```python
from build123d import *

# Parameters (mm, degrees)
SKETCH_1_R                       = 4
EXTRUDE_1_DEPTH                  = 41.5
HOLE_WIZARD_M4_1_D               = 3.3
HOLE_WIZARD_M4_1_DEPTH           = 12.1
HOLE_WIZARD_M4_1_TIP             = 0.991420021
HOLE_WIZARD_M4_1_ON_FACE_2_D     = 3.3
HOLE_WIZARD_M4_1_ON_FACE_2_DEPTH = 12.1
HOLE_WIZARD_M4_1_ON_FACE_2_TIP   = 0.991420021
CHAMFER_1_SIZE                   = 0.5
SKETCH_3_R                       = 2.5
EXTRUDE_1_2_DEPTH                = 6
CHAMFER_2_SIZE                   = 0.5
SKETCH_4_OUTSIDE_W               = 27.944
SKETCH_4_OUTSIDE_H               = 27.944
SKETCH_4_OUTSIDE_W_2             = 7
SKETCH_4_OUTSIDE_H_2             = 10.356925226
CUT_EXTRUDE_1_DEPTH              = 10


with BuildPart() as part:
    # 草图1 → Extrude 1 (new, symmetric)
    with BuildSketch(Plane.XY):
        Circle(SKETCH_1_R)
    extrude(amount=EXTRUDE_1_DEPTH, both=True)

    # M4 螺纹孔1
    with Locations(Plane.XY.offset(41.5)):
        with Locations((0, 0)):
            Hole(HOLE_WIZARD_M4_1_D / 2, depth=HOLE_WIZARD_M4_1_DEPTH)
            with Locations((0, 0, -(HOLE_WIZARD_M4_1_DEPTH + HOLE_WIZARD_M4_1_TIP / 2))):  # 118° drill point
                Cone(0, HOLE_WIZARD_M4_1_D / 2, HOLE_WIZARD_M4_1_TIP, mode=Mode.SUBTRACT)

    # M4 螺纹孔1 on face 2
    with Locations(Plane(origin=(0, 0, -41.5), x_dir=(-1, 0, 0), z_dir=(0, 0, -1))):
        with Locations((0, 0)):
            Hole(HOLE_WIZARD_M4_1_ON_FACE_2_D / 2, depth=HOLE_WIZARD_M4_1_ON_FACE_2_DEPTH)
            with Locations((0, 0, -(HOLE_WIZARD_M4_1_ON_FACE_2_DEPTH + HOLE_WIZARD_M4_1_ON_FACE_2_TIP / 2))):  # 118° drill point
                Cone(0, HOLE_WIZARD_M4_1_ON_FACE_2_D / 2, HOLE_WIZARD_M4_1_ON_FACE_2_TIP, mode=Mode.SUBTRACT)

    # 倒角1
    chamfer_1_edges = [part.edges().sort_by_distance(p)[0] for p in [
        (-4, 0, -41.5),
        (-4, 0, 41.5),
        (-1.65, 0, -41.5),
        (1.65, 0, 41.5),
    ]]
    chamfer(chamfer_1_edges, length=CHAMFER_1_SIZE)

    # 草图3 → Extrude 1 2 (add)
    with BuildSketch(Plane(origin=(0, 0, -41.5), x_dir=(-1, 0, 0), z_dir=(0, 0, -1))):
        with Locations(Location((0, 0, 0), (0, 0, 180))):
            Circle(SKETCH_3_R)
    extrude(amount=EXTRUDE_1_2_DEPTH)

    # 倒角2
    chamfer_2_edges = [part.edges().sort_by_distance(p)[0] for p in [
        (-2.5, 0, -47.5),
    ]]
    chamfer(chamfer_2_edges, length=CHAMFER_2_SIZE)

    # 草图4 outside → 切除-拉伸1 (cut)
    with BuildSketch(Plane(origin=(0, 0, -41.5), x_dir=(-1, 0, 0), z_dir=(0, 0, -1))):
        Rectangle(SKETCH_4_OUTSIDE_W, SKETCH_4_OUTSIDE_H)
        Rectangle(SKETCH_4_OUTSIDE_W_2, SKETCH_4_OUTSIDE_H_2, mode=Mode.SUBTRACT)
    extrude(amount=-CUT_EXTRUDE_1_DEPTH, mode=Mode.SUBTRACT)


solid = part.part
```
Check sheet for the modelled part. Datum: model origin and axes. Units: mm. A direction names the side the tool comes from. Give positions to 0.01 mm unless a question says otherwise; leave off trailing zeros. Write each loop counter-clockwise with the first axis right and the second up, starting at its lowest first coordinate (ties: lowest second). Pieces come first, ordered by that corner, then holes. Notation, with made-up numbers: (42.25, 50.25) -> (70.25, 50.25) arc R13 cw to (70.25, 64.25) -> close; hole circle Ø3 at (17, -36.75). An arc over 180 degrees is marked (long way). Use CSV: the item, a comma, the result in double quotes. Start each with the question number.
Q1. Tool access check on faces 1 (the flat face through (2, -2, -41.5)), 2 (the conical face through (0.1, -0.3, -28.6)), 3 (the cylindrical face through (1.216, 1.115, 35.119)), 4 (the flat face through (3.5, 0, -37)), 5 (the flat face through (-3.5, 0, -37)). Record the directions out of +Z, -Z, +X, -X, +Y, -Y that give a thin tool (end or side, any length) a straight path to the whole face; none if there is none.
Q2. Scan lines: line 1 along Y through (x, z) = (0, -32.25); line 2 along Z through (x, y) = (-0.5, -2.75); line 3 along Z through (x, y) = (1.75, -0.5). Record each from-to range of solid material in increasing order.
Q3. Cross-section at A-A on z = -33. Enter the section's corners in (x, y).
Q4. Cross-section at B-B on z = -6. Enter the section's corners in (x, y), and give its area (3 significant figures).
Q5. Depth check by flat-ended pin: P1, Ø1.2, axis at y = 0, z = -34.5, coming from the +X side; P2, Ø1.5, axis at y = -1, z = 16, coming from the -X side; P3, Ø2, axis at x = -1, y = 0, coming from the +Z side. Enter the tip coordinate at first touch or a pass-through.
Q6. Release check for a two-part mould opening along Z. For faces 6 (the cylindrical face through (-2.5, -0.1, -44.2)), 7 (the flat face through (0, 0, -47.5)), 8 (the cylindrical face through (-1.216, 1.115, -35.119)) record: +Z half, -Z half, draft (parallel to the pull), parting line (faces both ways), or undercut.
Working result:
1,face 1,"-Z"
1,face 2,"none"
1,face 3,"+Z"
1,face 4,"-Z, +X, +Y, -Y"
1,face 5,"-Z, -X, +Y, -Y"
2,line 1,"y = -4 to -1.65, 1.65 to 4"
2,line 2,"z = -41.5 to 41.5"
2,line 3,"z = -47.5 to -41.5, -41.17 to 41.17"
3,outline,"(-3.5, -1.94) arc R4 ccw to (3.5, -1.94) -> (3.5, 1.94) arc R4 ccw to (-3.5, 1.94) -> close; hole circle Ø3.3 at (0, 0)"
4,outline,"circle Ø8 at (0, 0)"
4,area,"50.3 mm^2"
5,P1,"stops at x = 3.5"
5,P2,"stops at x = -3.99"
5,P3,"stops at z = 41.35"
6,face 6,"draft"
6,face 7,"-Z half"
6,face 8,"undercut"
